Autodesk Inventor part; units mm, degrees
ref_plane "YZ Plane" through (0, 0, 0) normal (1, 0, 0) x (0, 1, 0)
ref_plane "XZ Plane" through (0, 0, 0) normal (0, 1, 0) x (-1, 0, 0)
ref_plane "XY Plane" through (0, 0, 0) normal (0, 0, 1) x (1, 0, 0)
sketch "Sketch1" plane through (0, 0, 0) normal (0, 0, 1) x (1, 0, 0)
  line L0 (2.8868, 0) -> (1.4434, -2.5)
  line L1 (1.4434, -2.5) -> (-1.4434, -2.5)
  line L2 (-1.4434, -2.5) -> (-2.8868, 0)
  line L3 (-2.8868, 0) -> (-1.4434, 2.5)
  line L4 (-1.4434, 2.5) -> (1.4434, 2.5)
  line L5 (1.4434, 2.5) -> (2.8868, 0)
  point P0 (0, 0)
  point P1 (0, 0)
  dimension "d0" = 5
extrude "Extrusion1" add sketch "Sketch1" along normal blind 7
sketch "Sketch2" plane through (0, 0, 7) normal (0, 0, 1) x (1, 0, 0)
  circle A0 centre (0, 0) radius 1.5
  dimension "d3" = 3
extrude "Extrusion2" add sketch "Sketch2" along normal blind 8
sketch "Sketch3" plane through (0, 0, 0) normal (0, 0, -1) x (-1, 0, 0)
  circle A0 centre (0, 0) radius 1.5
  dimension "d6" = 3
extrude "Extrusion3" cut sketch "Sketch3" against normal blind 4
properties part number "Spacer7mm_m3"
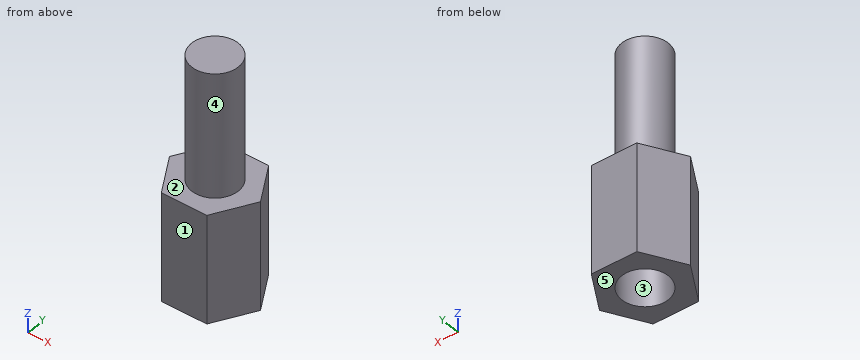
For this review, take the finished solid that the model builds, in its own axes (mm). Face numbers are marked on the shaded views. A direction names the side the tool comes from. Give positions to 0.01 mm unless a question says otherwise; leave off trailing zeros. Write each loop counter-clockwise with the first axis right and the second up, starting at its lowest first coordinate (ties: lowest second). Pieces come first, ordered by that corner, then holes.
Item 1: Insertion check: P1, Ø3, axis at x = -1, z = 11.5, coming from the +Y side; P2, Ø1.5, axis at y = -0.5, z = 11, coming from the +X side; P3, Ø1, axis at y = 2, z = 6.5, coming from the +X side. Each pin has a flat end and moves straight along its axis. Give the tip position at first contact, or say it passes through.
Item 2: Machinability: for the marked faces 4 and 5, which of the approach directions +Z, -Z, +X, -X, +Y, -Y give a long, thin tool a straight path to every point of the face, cutting with its end or side? Answer none if there is none.
Item 3: Wall thickness on probe 1 along Y at (x, z) = (0, 1.95); probe 2 along Z at (x, y) = (1.8, -1.35); probe 3 along Z at (x, y) = (0.3, -1.15): over which ranges is each line inside the solid? List them lowest first.
Item 4: Take a section at A-A (x = 0). Give the boundary of the cut face in (y, z), and give its area (3 significant figures).
Item 5: Take a section at B-B (z = 4.25). Give the boundary of the cut face in (x, y), and give its area (3 significant figures).
Item 6: The part is to be moulded in two halves that separate along Y. For the marked faces 1, 2 and 3, say which applies: +Y half, -Y half, draft (parallel to the pull), parting line (faces both ways), or undercut.
Item 7: Take a section at D-D (z = 8.25). Give the boundary of the cut face in (x, y).
Item 8: Take a section at C-C (y = 0.4). Give the boundary of the cut face in (x, z), and give its area (3 significant figures).
Established:
1. P1: stops at y = 1.5
1. P2: stops at x = 1.5
1. P3: stops at x = 2.02
2. face 4: +Z
2. face 5: -Z, +X, -X, +Y, -Y
3. probe 1: y = -2.5 to -1.5, 1.5 to 2.5
3. probe 2: z = 0 to 7
3. probe 3: z = 4 to 15
4. outline: (-2.5, 0) - (-1.5, 0) - (-1.5, 4) - (1.5, 4) - (1.5, 0) - (2.5, 0) - (2.5, 7) - (1.5, 7) - (1.5, 15) - (-1.5, 15) - (-1.5, 7) - (-2.5, 7) - close
4. area: 47.0 mm2
5. outline: (-2.89, 0) - (-1.44, -2.5) - (1.44, -2.5) - (2.89, 0) - (1.44, 2.5) - (-1.44, 2.5) - close
5. area: 21.7 mm2
6. face 1: -Y half
6. face 2: draft
6. face 3: undercut
7. outline: circle Ø3 at (0, 0)
8. outline: (-2.66, 0) - (-1.45, 0) - (-1.45, 4) - (1.45, 4) - (1.45, 0) - (2.66, 0) - (2.66, 7) - (1.45, 7) - (1.45, 15) - (-1.45, 15) - (-1.45, 7) - (-2.66, 7) - close
8. area: 48.7 mm2
